Can you work these out from the drawing? Everything is in mm from the part's minimum corner. Coordinates: 2 decimals unless noted, no trailing zeros. Loops run counter-clockwise (first coordinate to the right, second up) from the corner with the lowest first, then second, coordinate; pieces in that order, holes last.
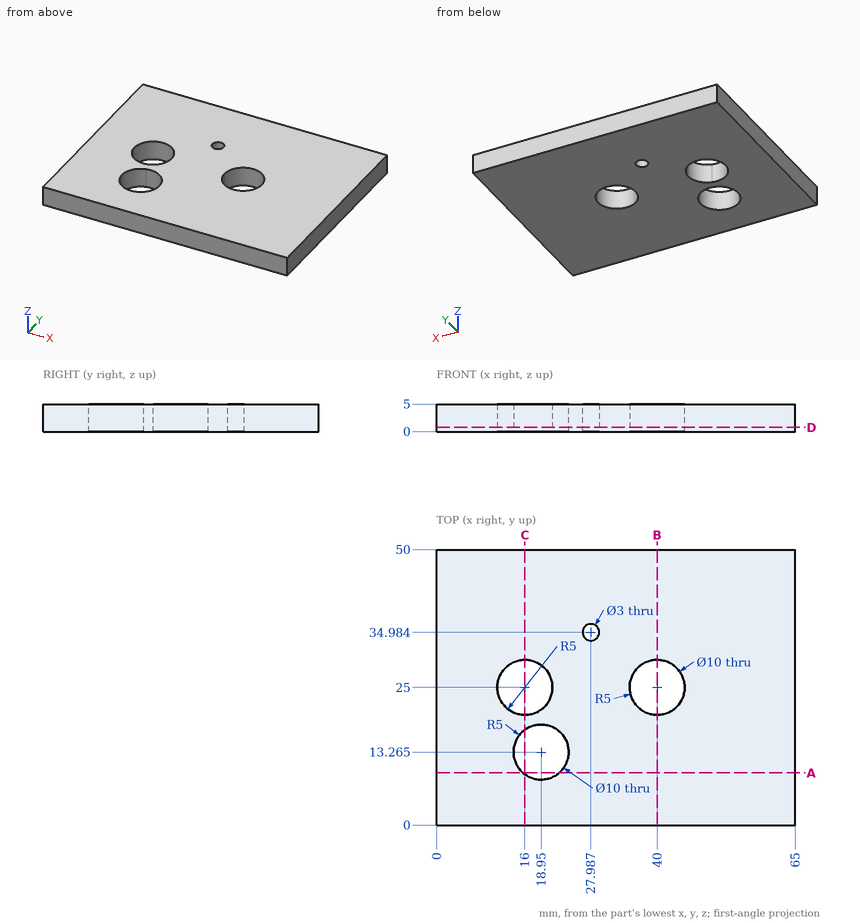
(1) I need wall thicknesses on probe 1 along X at (y, z) = (25, 2.65); probe 2 along X at (y, z) = (26, 2.65); probe 3 along Y at (x, z) = (18, 2.9) (1 decimal). Which ranges of each line are inside material? Lowest first, please.
Answers:
probe 1: x = 0 to 11, 21 to 35, 45 to 65
probe 2: x = 0 to 11.1, 20.9 to 35.1, 44.9 to 65
probe 3: y = 0 to 8.4, 18.2 to 20.4, 29.6 to 50
(2) Imagine slicing it at B-B, the plane x = 40. Write out the boundary of the cut face in (y, z).
Answers:
outline: (0, 0) - (20, 0) - (20, 5) - (0, 5) - close; (30, 0) - (50, 0) - (50, 5) - (30, 5) - close
(3) Imagine slicing it at A-A, the plane y = 9.5. Write out the boundary of the cut face in (x, z), and give its area (3 significant figures).
Answers:
outline: (0, 0) - (15.66, 0) - (15.66, 5) - (0, 5) - close; (22.24, 0) - (65, 0) - (65, 5) - (22.24, 5) - close
area: 292 mm2
(4) Imagine slicing it at D-D, the plane z = 0.75. State how many separate pieces and enclosed holes the cut face has, and give its area (3 significant figures).
Answers:
separate pieces: 1
enclosed holes: 4
area: 3,010 mm2
(5) Imagine slicing it at C-C, the plane x = 16. Write out the boundary of the cut face in (y, z), and give its area (3 significant figures).
Answers:
outline: (0, 0) - (9.23, 0) - (9.23, 5) - (0, 5) - close; (17.3, 0) - (20, 0) - (20, 5) - (17.3, 5) - close; (30, 0) - (50, 0) - (50, 5) - (30, 5) - close
area: 160 mm2
